Here's how the part is built. I have some questions about the finished solid (model axes, mm). A direction names the side the tool comes from. Round coordinates to 2 decimals unless told otherwise and drop trailing zeros. Write each loop counter-clockwise with the first axis right and the second up, starting at its lowest first coordinate (ties: lowest second). Pieces come first, ordered by that corner, then holes. Notation, with made-up numbers: (59, 14.5) -> (84, 14.5) arc R11 ccw to (84, 19.5) -> close; hole circle Ø9 at (59.25, 13). An arc over 180 degrees is marked (long way). Answer in a Markdown table with one row per item.
from build123d import *

# Parameters (mm, degrees)
F0_W     = 30
F0_H     = 20
F1_DEPTH = 0.5
F2_D     = 1.5
F2_DEPTH = 0.501


with BuildPart() as f1:
    # F0 (on Front) → F1 (new body, symmetric)
    with BuildSketch(Plane.XZ):
        Rectangle(F0_W, F0_H)
    extrude(amount=F1_DEPTH, both=True)

    # F2 (through all, one way)
    with BuildSketch(Plane(origin=(0, 0, 0), x_dir=(1, 0, 0), z_dir=(0, 1, 0))):
        with Locations((-12, -5), (12, -5), (7.75, 5), (-7.75, 5)):
            Circle(F2_D / 2)
    extrude(amount=-F2_DEPTH, mode=Mode.SUBTRACT)


solid = f1.part
1) For pin 1 (1.2 mm diameter, centred on x = 7.75, z = -5, fed in from -Y), with a flat end and sliding along its axis, tell me the tip position at first contact or that it passes through.
Response:
| item | result |
|---|---|
| pin 1 | stops at y = 0 |
2) Which directions (+Z, -Z, +X, -X, +Y, -Y) give clear straight access to the entire face, cutting with the end or side of a thin tool? Please do faces 1 (the face through (0, 0, -10)), 2 (the face through (-8, 0, -5)).
Response:
| item | result |
|---|---|
| face 1 | -Z, +X, -X, +Y, -Y |
| face 2 | -Y |
3) I want a section at B-B, the plane x = 7.75. List the corners of the cut face in (y, z) for me.
Response:
| item | result |
|---|---|
| outline | (-0.5, -10) -> (0.5, -10) -> (0.5, 10) -> (-0.5, 10) -> (-0.5, -4.25) -> (0, -4.25) -> (0, -5.75) -> (-0.5, -5.75) -> close |
4) I want a section at A-A, the plane z = -5. List the corners of the cut face in (x, y) for me, and give its area (3 significant figures).
Response:
| item | result |
|---|---|
| outline | (-15, -0.5) -> (-8.5, -0.5) -> (-8.5, 0) -> (-7, 0) -> (-7, -0.5) -> (7, -0.5) -> (7, 0) -> (8.5, 0) -> (8.5, -0.5) -> (15, -0.5) -> (15, 0.5) -> (-15, 0.5) -> close |
| area | 28.5 mm^2 |
5) I need wall thicknesses on line 1 (X direction, y = -0.4, z = 5); line 2 (Z direction, x = 12, y = -0.2); line 3 (Z direction, x = 7.75, y = -0.1). Which ranges of each line are inside material? Lowest first, please. Write a range as [from, to].
Response:
| item | result |
|---|---|
| line 1 | x = [-15, -12.75], [-11.25, 11.25], [12.75, 15] |
| line 2 | z = [-10, 4.25], [5.75, 10] |
| line 3 | z = [-10, -5.75], [-4.25, 10] |
